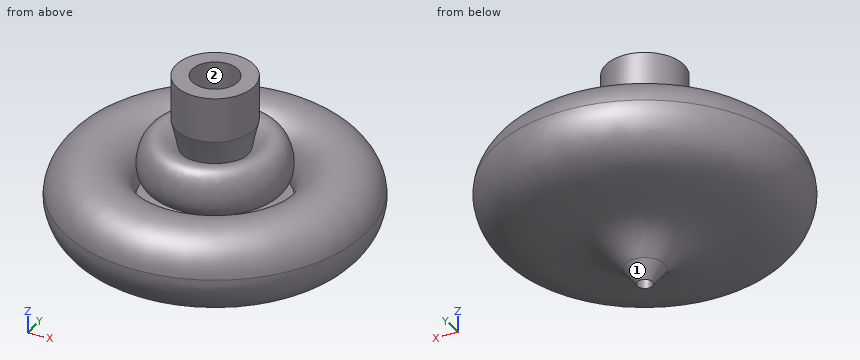
```python
from build123d import *

# Parameters (mm, degrees)
F2_R     = 4.7625
F3_DEPTH = 9.525
F4_R     = 1.583755089
F5_DEPTH = 19.05


with BuildPart() as f1:
    # F0 (on Front) → F1 (revolve)
    with BuildSketch(Plane.XZ):
        with BuildLine():
            Line((0, 46.8931338228), (0, 0))
            Line((0, 0), (4.0591530134, 5.2044031537))
            add(Edge.make_bspline(
                [(31.4793007411, 22.2346165378), (31.8463772185, 20.4411681612), (29.5054120617, 11.2492719757), (11.8885656035, 11.5250736881), (6.6367846724, 8.350135012), (4.0591530134, 5.2044031537)],
                knots=[0.5345439542, 0.5345439542, 0.5345439542, 0.5345439542, 0.6486193958, 0.8457425586, 1, 1, 1, 1], degree=3))
            add(Edge.make_bspline(
                [(14.6243430234, 20.5337022678), (17.3788808913, 20.130808601), (24.9437703638, 20.5617479815), (30.444556084, 24.7173182926), (31.3930745838, 22.6558970375), (31.4793007411, 22.2346165378)],
                knots=[0.2746906864, 0.2746906864, 0.2746906864, 0.2746906864, 0.369317623, 0.5077476664, 0.5345439542, 0.5345439542, 0.5345439542, 0.5345439542], degree=3))
            add(Edge.make_bspline(
                [(8.1183060268, 23.4465669114), (9.4978348292, 21.8910995306), (11.9068224974, 20.9311815771), (14.6243430234, 20.5337022678)],
                knots=[0.1813354106, 0.1813354106, 0.1813354106, 0.1813354106, 0.2746906864, 0.2746906864, 0.2746906864, 0.2746906864], degree=3))
            add(Edge.make_bspline(
                [(6.8602322526, 31.9419862034), (6.2722594814, 28.4500390964), (6.3389179378, 25.4528897408), (8.1183060268, 23.4465669114)],
                knots=[0.0609209143, 0.0609209143, 0.0609209143, 0.0609209143, 0.1813354106, 0.1813354106, 0.1813354106, 0.1813354106], degree=3))
            add(Edge.make_bspline(
                [(8.1183060268, 37.5577078759), (7.6227351887, 35.6019744349), (7.1577034033, 33.7086556398), (6.8602322526, 31.9419862034)],
                knots=[0, 0, 0, 0, 0.0609209143, 0.0609209143, 0.0609209143, 0.0609209143], degree=3))
            Line((8.1183060268, 37.5577078759), (8.1183060268, 46.8931338228))
            Line((8.1183060268, 46.8931338228), (0, 46.8931338228))
        make_face()
        with BuildLine():
            add(Edge.make_bspline(
                [(14.6243430234, 20.5337022678), (17.3788808913, 20.130808601), (24.9437703638, 20.5617479815), (30.444556084, 24.7173182926), (31.3930745838, 22.6558970375), (31.4793007411, 22.2346165378)],
                knots=[0.2746906864, 0.2746906864, 0.2746906864, 0.2746906864, 0.369317623, 0.5077476664, 0.5345439542, 0.5345439542, 0.5345439542, 0.5345439542], degree=3))
            ThreePointArc((31.4793007411, 22.2346165378), (22.2369207101, 29.4593017204), (14.6243430234, 20.5337022678))
        make_face()
        with BuildLine():
            add(Edge.make_bspline(
                [(6.8602322526, 31.9419862034), (9.9612760445, 34.8264937244), (14.3434078349, 34.0282924349), (15.4421353586, 22.9271029088), (8.7709869873, 24.4450941789), (8.1183060268, 23.4465669114)],
                knots=[0.0076568861, 0.0076568861, 0.0076568861, 0.0076568861, 0.338323865, 0.6963180309, 1, 1, 1, 1], degree=3))
            add(Edge.make_bspline(
                [(6.8602322526, 31.9419862034), (6.2722594814, 28.4500390964), (6.3389179378, 25.4528897408), (8.1183060268, 23.4465669114)],
                knots=[0.0609209143, 0.0609209143, 0.0609209143, 0.0609209143, 0.1813354106, 0.1813354106, 0.1813354106, 0.1813354106], degree=3))
        make_face()
    revolve(axis=Axis((0, 0, 23.4465669114), (0, 0, -1)))

    # F2 (on face) → F3 (cut)
    with BuildSketch(Plane.XY.offset(46.8931338228)):
        Circle(F2_R)
    extrude(amount=-F3_DEPTH, mode=Mode.SUBTRACT)

    # F4 (on Top) → F5 (cut)
    with BuildSketch(Plane.XY):
        Circle(F4_R)
    extrude(amount=F5_DEPTH, mode=Mode.SUBTRACT)


solid = f1.part
```
Source: CAD feature listing. Evaluate the final solid. Frame: model axes, mm. Face numbers are marked on the shaded views. A direction names the side the tool comes from. Give positions to 0.01 mm unless a question says otherwise; leave off trailing zeros. Order: outer loops, then holes, each group sorted by start corner. A loop starts at its lowest first (then second) coordinate and runs counter-clockwise, first axis right, second up. Notation, with made-up numbers: (-1, 18) -> (11, 18) arc R19 cw to (11, 50) -> close; hole circle Ø1 at (-8.75, -12). An arc over 180 degrees is marked (long way). Use a Markdown table: item, result.
Q1. Access query for the marked faces 1 and 2. Directions: +Z, -Z, +X, -X, +Y, -Y. A direction counts if a zero-diameter tool reaches every point of the face in a straight line with its end or side. Return the directions, or none.
A:
| item | result |
|---|---|
| face 1 | -Z |
| face 2 | +Z |
Q2. Material intervals for line 1 (Y direction, x = 0, z = 41.25); line 2 (Y direction, x = 0, z = 14.5); line 3 (Y direction, x = 6, z = 32.5), sorted ascending. Write a range as [from, to].
A:
| item | result |
|---|---|
| line 1 | [-8.12, -4.76], [4.76, 8.12] |
| line 2 | [-28.35, -1.58], [1.58, 28.35] |
| line 3 | [-11.89, -4.49], [-3.52, 3.52], [4.49, 11.89] |
Q3. Section A-A (z = 41). Return the cut outline in (x, y) (1 decimal), and give its area (3 significant figures).
A:
| item | result |
|---|---|
| outline | circle Ø16.2 at (0, 0); hole circle Ø9.5 at (0, 0) |
| area | 136 mm^2 |
Q4. First-contact query: P1, Ø4, axis at x = 0, y = 0, coming from the +Z side; P2, Ø10, axis at y = 15, z = 8.5, coming from the -X side; P3, Ø2.5, axis at x = 0, y = 0.5, coming from the -Z side; P4, Ø5, axis at x = -15.5, y = -18, coming from the -Z side. Flat tips, straight axial feed; report the tip coordinate or a pass-through.
A:
| item | result |
|---|---|
| P1 | z = 37.37 |
| P2 | x = -22.73 |
| P3 | z = 2.03 |
| P4 | z = 11.7 |
